Work out the finished part from the listing and answer in its coordinate system (mm). Face numbers are marked on the shaded views. A direction names the side the tool comes from. Round coordinates to 2 decimals unless told otherwise and drop trailing zeros. Write each loop counter-clockwise with the first axis right and the second up, starting at its lowest first coordinate (ties: lowest second). Pieces come first, ordered by that corner, then holes. Notation, with made-up numbers: M 43,86.25 L 77,86.25 A22 ccw 77,107.25 Z; hole C 72,17 d11. An arc over 180 degrees is marked long. Answer in a Markdown table with one row per item.
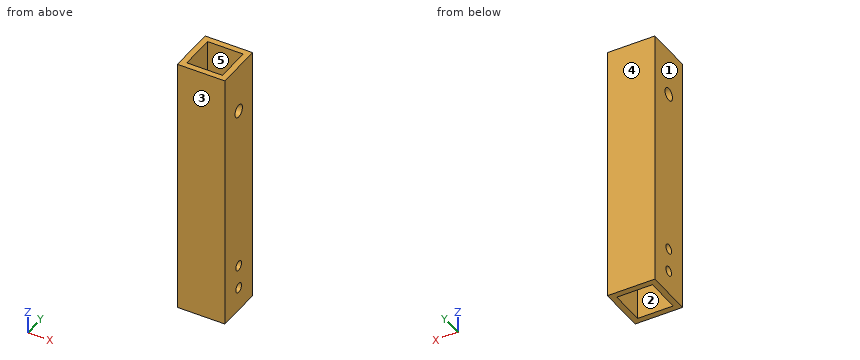
Autodesk Inventor part; units mm, degrees
ref_plane "YZ Plane" through (0, 0, 0) normal (1, 0, 0) x (0, 1, 0)
ref_plane "XZ Plane" through (0, 0, 0) normal (0, 1, 0) x (-1, 0, 0)
ref_plane "XY Plane" through (0, 0, 0) normal (0, 0, 1) x (1, 0, 0)
sketch "Sketch1" plane through (0, 0, 0) normal (0, 0, 1) x (1, 0, 0)
  line L0 (-12.7, -12.7) -> (12.7, -12.7)
  line L1 (12.7, -12.7) -> (12.7, 12.7)
  line L2 (12.7, 12.7) -> (-12.7, 12.7)
  line L3 (-12.7, 12.7) -> (-12.7, -12.7)
  line L4 (-12.7, -12.7) -> (12.7, 12.7) construction
  line L5 (12.7, -12.7) -> (-12.7, 12.7) construction
  line L6 (-9.525, 9.525) -> (9.525, 9.525)
  line L7 (9.525, 9.525) -> (9.525, -9.525)
  line L8 (9.525, -9.525) -> (-9.525, -9.525)
  line L9 (-9.525, -9.525) -> (-9.525, 9.525)
  point P0 (0, 0)
  dimension "width" = 25.4
  dimension "height" = 25.4
  dimension "thickness" = 3.175
extrude "Extrusion1" add sketch "Sketch1" along normal mid plane 139.7
sketch "Sketch2" plane through (12.7, -12.7, 69.85) normal (1, 0, 0) x (0, 0, -1)
  line L0 (0, 0) -> (0, 25.4) construction
  point P0 (69.85, 12.7)
  point P1 (25.4, 12.7)
  dimension "d5" = 25.4
hole "Hole1" at (12.7, 0, 44.45) direction (-1, 0, 0) diameter 6.7564 end through all
sketch "Sketch3" plane through (12.7, -12.7, 69.85) normal (1, 0, 0) x (0, 0, -1)
  line L0 (139.7, 25.4) -> (139.7, 0) construction
  point P0 (69.85, 12.7)
  point P1 (127, 12.7)
  point P2 (114.3, 12.7)
  point P3 (139.7, 12.7)
  dimension "d13" = 12.7
  dimension "d14" = 12.7
hole "Hole2" at (12.7, 0, -57.15) at (12.7, 0, -44.45) direction (-1, 0, 0) diameter 5.1054 end through all
properties part number "CHD-003" material "Aluminum 6061"
1. The part is cut by section A-A (x = 5.25). Determine the outline of the cut face in (y, z) (3 decimals), plus the area to 3 significant figures.
Calculated:
| item | result |
|---|---|
| outline | M -12.7,-69.85 L -9.525,-69.85 L -9.525,69.85 L -12.7,69.85 Z; M 9.525,-69.85 L 12.7,-69.85 L 12.7,69.85 L 9.525,69.85 Z |
| area | 887 mm² |
2. The part is cut by section C-C (z = 44.45). Determine the outline of the cut face in (x, y) (3 decimals), plus the area to 3 significant figures.
Calculated:
| item | result |
|---|---|
| outline | M -12.7,-12.7 L 12.7,-12.7 L 12.7,-3.378 L 9.525,-3.378 L 9.525,-9.525 L -9.525,-9.525 L -9.525,-3.378 L -12.7,-3.378 Z; M -12.7,3.378 L -9.525,3.378 L -9.525,9.525 L 9.525,9.525 L 9.525,3.378 L 12.7,3.378 L 12.7,12.7 L -12.7,12.7 Z |
| area | 239 mm² |
3. Determine the mould class of the marked faces 3, 4 and 5 for opening direction Y: released by +Y, released by -Y, zero draft, split by the parting line, or undercut.
Calculated:
| item | result |
|---|---|
| face 3 | released by -Y |
| face 4 | released by +Y |
| face 5 | undercut |
4. A tool of negligible diameter and unlimited length cuts with its end or side. For the marked faces 1 and 2, from which of +Z, -Z, +X, -X, +Y, -Y can it reach the whole face along a straight path? Write none if from no direction.
Calculated:
| item | result |
|---|---|
| face 1 | +Z, -Z, -X, +Y, -Y |
| face 2 | +Z, -Z |
5. Consider line 1 along Z through (x, y) = (-11.6, 0); line 2 along X through (y, z) = (4.25, 55.5) (3 decimals). Determine where each line is inside the solid, lowest interval first. Write a range as from..to.
Calculated:
| item | result |
|---|---|
| line 1 | z = -69.85..-59.7, -54.6..-47, -41.9..41.07, 47.83..69.85 |
| line 2 | x = -12.7..-9.525, 9.525..12.7 |
6. The part is cut by section D-D (z = 59). Determine the outline of the cut face in (x, y) (3 decimals), plus the area to 3 significant figures.
Calculated:
| item | result |
|---|---|
| outline | M -12.7,-12.7 L 12.7,-12.7 L 12.7,12.7 L -12.7,12.7 Z; hole M -9.525,-9.525 L 9.525,-9.525 L 9.525,9.525 L -9.525,9.525 Z |
| area | 282 mm² |
